The figure shows three views and two pictorial views of one solid part (mm, origin at its lowest corner). Answer the questions. A direction names the side the tool comes from. Round coordinates to 2 decimals unless told otherwise and drop trailing zeros. Order: outer loops, then holes, each group sorted by start corner. A loop starts at its lowest first (then second) coordinate and runs counter-clockwise, first axis right, second up.
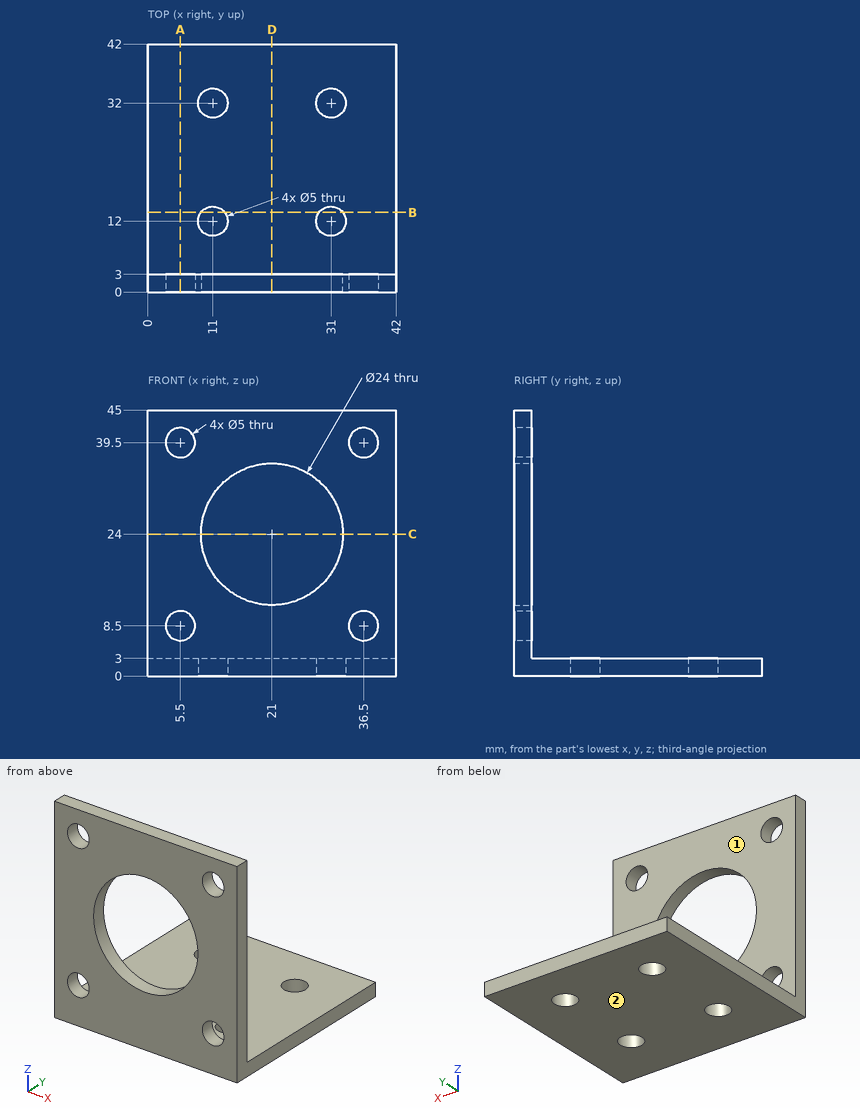
Item 1: Find section D-D (x = 21). Write down the section's boundary in (y, z), plus the area to 3 significant figures.
Item 2: Given pin 1 (1.5 mm diameter, centred on x = 29.5, y = 25.5, fed in from +Z); pin 2 (6.5 mm diameter, centred on x = 36.5, z = 8.5, fed in from +Y), each flat-ended and moving along its own axis, determine where each tip first touches the part or whether it passes through.
Item 3: Find the intervals of material crossed by line 1 along Y through (x, z) = (11, 1.9); line 2 along Z through (x, y) = (36.5, 2.15); line 3 along Y through (x, z) = (15, 8.5), in increasing order.
Item 4: A tool of negligible diameter and unlimited length cuts with its end or side. For the marked faces 1 and 2, from which of +Z, -Z, +X, -X, +Y, -Y can it reach the whole face along a straight path? Write none if from no direction.
Item 5: Find section A-A (x = 5.5). Write down the section's boundary in (y, z).
Item 6: Find section B-B (y = 13.5). Write down the section's boundary in (x, z), plus the area to 3 significant figures.
Item 7: Find section C-C (z = 24). Write down the section's boundary in (x, y), plus the area to 3 significant figures.
Model answer:
1. outline: (0, 0) - (42, 0) - (42, 3) - (3, 3) - (3, 12) - (0, 12) - close; (0, 36) - (3, 36) - (3, 45) - (0, 45) - close
1. area: 180 mm2
2. pin 1: stops at z = 3
2. pin 2: stops at y = 3
3. line 1: y = 0 to 9.5, 14.5 to 29.5, 34.5 to 42
3. line 2: z = 0 to 6, 11 to 37, 42 to 45
3. line 3: y = 0 to 3
4. face 1: +Z, +X, -X, +Y
4. face 2: -Z, +X, -X, +Y, -Y
5. outline: (0, 0) - (42, 0) - (42, 3) - (3, 3) - (3, 6) - (0, 6) - close; (0, 11) - (3, 11) - (3, 37) - (0, 37) - close; (0, 42) - (3, 42) - (3, 45) - (0, 45) - close
6. outline: (0, 0) - (9, 0) - (9, 3) - (0, 3) - close; (13, 0) - (29, 0) - (29, 3) - (13, 3) - close; (33, 0) - (42, 0) - (42, 3) - (33, 3) - close
6. area: 102 mm2
7. outline: (0, 0) - (9, 0) - (9, 3) - (0, 3) - close; (33, 0) - (42, 0) - (42, 3) - (33, 3) - close
7. area: 54.0 mm2
